Autodesk Fusion 360 part; units mm, degrees
sketch "Esquisse1" plane through (0, 0, 0) normal (0, 1, 0) x (1, 0, 0)
  circle A0 centre (0, 0) radius 18.15
  circle A1 centre (0, 0) radius 15.5
  dimension "d1" = 36.3
  dimension "d2" = 31
extrude "Extrusion1" add sketch "Esquisse1" along normal blind 10 makes body 1
sketch "Esquisse2" plane through (0, 10, 0) normal (0, 1, 0) x (-1, 0, 0)
  circle A0 centre (0, 0) radius 15.5
  circle A1 centre (0, 0) radius 18.15
  circle A2 centre (0, 0) radius 25
  dimension "d5" = 50
extrude "Extrusion2" add sketch "Esquisse2" along normal blind 2 contours A1 | A2 bodies 1
sketch "Esquisse3" plane through (0, 0, 0) normal (0, 1, 0) x (1, 0, 0)
  circle A0 centre (0, 0) radius 16.65
  circle A1 centre (0, 0) radius 12.5
  dimension "d8" = 33.3
  dimension "d9" = 25
extrude "Extrusion3" add sketch "Esquisse3" along normal blind 5 bodies 1
sketch "Esquisse4" plane through (0, 12, 0) normal (0, 1, 0) x (-1, 0, 0)
  circle A0 centre (0, 0) radius 15.5
  circle A1 centre (0, 0) radius 25
  circle A2 centre (0, 0) radius 16.65
  circle A3 centre (0, 0) radius 10
  dimension "d12" = 33.3
  dimension "d13" = 20
extrude "Extrusion4" add sketch "Esquisse4" against normal blind 2 separate body contours A0 makes body 2
fillet "Congé1" radius 2 1 edges at (23.3082, 12, -9.0404) on bodies 1
sketch "Esquisse5" plane through (0, 12, 0) normal (0, 1, 0) x (-1, 0, 0)
  circle A0 centre (0, 0) radius 10
  circle A1 centre (0, 0) radius 15.5
  line L0 (0, 10.5) -> (1.9964, 13.9579)
  line L1 (0, 10.5) -> (3.9928, 10.5) construction
  line L2 (0, 10.5) -> (-2.0557, 13.9579)
  line L3 (-2.0557, 13.9579) -> (1.9964, 13.9579)
  line L4 (-6.1717, 8.4947) -> (-6.5891, 12.4657)
  line L5 (-9.8673, 10.0839) -> (-6.5891, 12.4657)
  line L6 (-6.1717, 8.4947) -> (-9.8673, 10.0839)
  line L7 (-9.9861, 3.2447) -> (-12.6578, 6.2119)
  line L8 (-13.91, 2.3582) -> (-12.6578, 6.2119)
  line L9 (-9.9861, 3.2447) -> (-13.91, 2.3582)
  line L10 (-9.9861, -3.2447) -> (-13.8917, -2.4145)
  line L11 (-12.6395, -6.2683) -> (-13.8917, -2.4145)
  line L12 (-9.9861, -3.2447) -> (-12.6395, -6.2683)
  line L13 (-6.1717, -8.4947) -> (-9.8194, -10.1187)
  line L14 (-6.5412, -12.5005) -> (-9.8194, -10.1187)
  line L15 (-6.1717, -8.4947) -> (-6.5412, -12.5005)
  line L16 (0, -10.5) -> (-1.9964, -13.9579)
  line L17 (2.0557, -13.9579) -> (-1.9964, -13.9579)
  line L18 (0, -10.5) -> (2.0557, -13.9579)
  line L19 (6.1717, -8.4947) -> (6.5891, -12.4657)
  line L20 (9.8673, -10.0839) -> (6.5891, -12.4657)
  line L21 (6.1717, -8.4947) -> (9.8673, -10.0839)
  line L22 (9.9861, -3.2447) -> (12.6578, -6.2119)
  line L23 (13.91, -2.3582) -> (12.6578, -6.2119)
  line L24 (9.9861, -3.2447) -> (13.91, -2.3582)
  line L25 (9.9861, 3.2447) -> (13.8917, 2.4145)
  line L26 (12.6395, 6.2683) -> (13.8917, 2.4145)
  line L27 (9.9861, 3.2447) -> (12.6395, 6.2683)
  line L28 (6.1717, 8.4947) -> (9.8194, 10.1187)
  line L29 (6.5412, 12.5005) -> (9.8194, 10.1187)
  line L30 (6.1717, 8.4947) -> (6.5412, 12.5005)
  dimension "d18" = 60
  dimension "d20" = 360
extrude "Extrusion5" cut sketch "Esquisse5" against normal blind 5 contours L0 L2 L3 | L4 L5 L6 | L7 L8 L9 | L10 L11 L12 | L13 L14 L15 | L16 L17 L18 | L19 L20 L21 | L22 L23 L24 | L25 L26 L27 | L28 L29 L30 bodies 2
combine "Combiner1" operation add target body 1 tool bodies 2
For this review, take the finished solid that the model builds, in its own axes (mm). A direction names the side the tool comes from. Coordinates: 2 decimals unless noted, no trailing zeros. Write each loop counter-clockwise with the first axis right and the second up, starting at its lowest first coordinate (ties: lowest second). Pieces come first, ordered by that corner, then holes. Notation, with made-up numbers: (45.5, 85.25) - (71.5, 85.25) arc R11 ccw to (71.5, 97.25) - close; hole circle Ø7 at (-5, 22.25). An arc over 180 degrees is marked (long way). Put each result on its own line as item: value.
1. Add section C-C, the plane y = 2. Give the boundary of the cut face in (x, z).
Values found:
outline: circle Ø36.3 at (0, 0); hole circle Ø25 at (0, 0)
2. Machinability: for faces 1 (the cylindrical face through (2.17, 11.01, -9.76)), 2 (the flat face through (-11.912, 11.014, 2.835)), which of the approach directions +Z, -Z, +X, -X, +Y, -Y give a long, thin tool a straight path to every point of the face, cutting with its end or side? Answer none if there is none.
Values found:
face 1: +Y, -Y
face 2: +Y
3. For pin 1 (4 mm diameter, centred on y = 5, z = 11, fed in from +X); pin 2 (6 mm diameter, centred on x = 6.5, y = 2, fed in from -Z); pin 3 (18 mm diameter, centred on x = 0, z = 0, fed in from -Y); pin 4 (1 mm diameter, centred on x = -5.5, y = 6.5, fed in from -Z), all flat-tipped, find the tip position at first contact; note any pin that passes through.
Values found:
pin 1: x = 15.76
pin 2: z = -17.81
pin 3: through
pin 4: z = -17.45
4. Mouldability with a two-part tool opening along Y and no side actions: class faces 3 (the flat face through (-17, 10, 8)), 4 (the cylindrical face through (-2.018, 7.465, 15.368)), 5 (the flat face through (13.257, 11.014, -4.368)) as released by +Y, released by -Y, zero draft, split by the parting line, or undercut.
Values found:
face 3: released by -Y
face 4: undercut
face 5: zero draft
5. Wall thickness on probe 1 along X at (y, z) = (3.35, 0); probe 2 along Z at (x, y) = (0, 7.1); probe 3 along Y at (x, z) = (-13.5, 1.5): over which ranges is each line inside the solid? List them lowest first.
Values found:
probe 1: -18.15 to -12.5, 12.5 to 18.15
probe 2: -18.15 to -15.5, 15.5 to 18.15
probe 3: 0 to 5, 10 to 12
6. Add section B-B, the plane y = 6.75. Give the boundary of the cut face in (x, z).
Values found:
outline: circle Ø36.3 at (0, 0); hole circle Ø31 at (0, 0)
